For this review, use the dimensioned drawing (mm, ordinates from the lowest corner) and the shaded views. A direction names the side the tool comes from. Coordinates: 2 decimals unless noted, no trailing zeros. Order: outer loops, then holes, each group sorted by start corner. A loop starts at its lowest first (then second) coordinate and runs counter-clockwise, first axis right, second up. Notation, with made-up numbers: (63, 79) -> (107, 79) arc R21 ccw to (107, 105) -> close; hole circle Ø3 at (0, 56). An arc over 180 degrees is marked (long way). Use one line per item in the form item = value. Start each with the question number.
(1) For the marked faces 1, 2 and 3, list the 3-axis set-ups (+Z, -Z, +X, -X, +Y, -Y) from which the entire face can be reached by the end or side of a thin tool; tool diameter is ignored.
(2) Take a section at C-C (y = 513.5). State the section outline as (x, z) points.
(3) Take a section at A-A (x = 444.5). State the section outline as (y, z) points, then the cut area to 3 significant figures.
(4) Wall thickness on line 1 along Y through (x, z) = (448, 212); line 2 along Y through (x, z) = (1625, 26) (1 decimal); line 3 along X through (y, z) = (483.5, 214) (1 decimal): over which ranges is each line inside the solid? List them lowest first.
(5) Take a section at D-D (x = 1898.5). State the section outline as (y, z) points (1 decimal), then the cut area to 3 significant figures.
(6) Insertion check: pin 1 Ø1.5 at (x, z) = (999.5, 161.5) entering from +Y; pin 2 Ø10 at (y, z) = (686, 196.5) entering from -X; pin 3 Ø1 at (y, z) = (616.5, 172.5) entering from -X. Each pin has a flat end and moves straight along its axis. Give the tip position at first contact, or say it passes through.
(7) Mouldability with a two-part tool opening along X and no side actions: class the marked faces 4, 5 and 6 as +X half, -X half, draft (parallel to the pull), parting line (faces both ways), or undercut.
(8) Take a section at B-B (z = 207). State the section outline as (x, y) points (1 decimal), then the cut area to 3 significant figures.
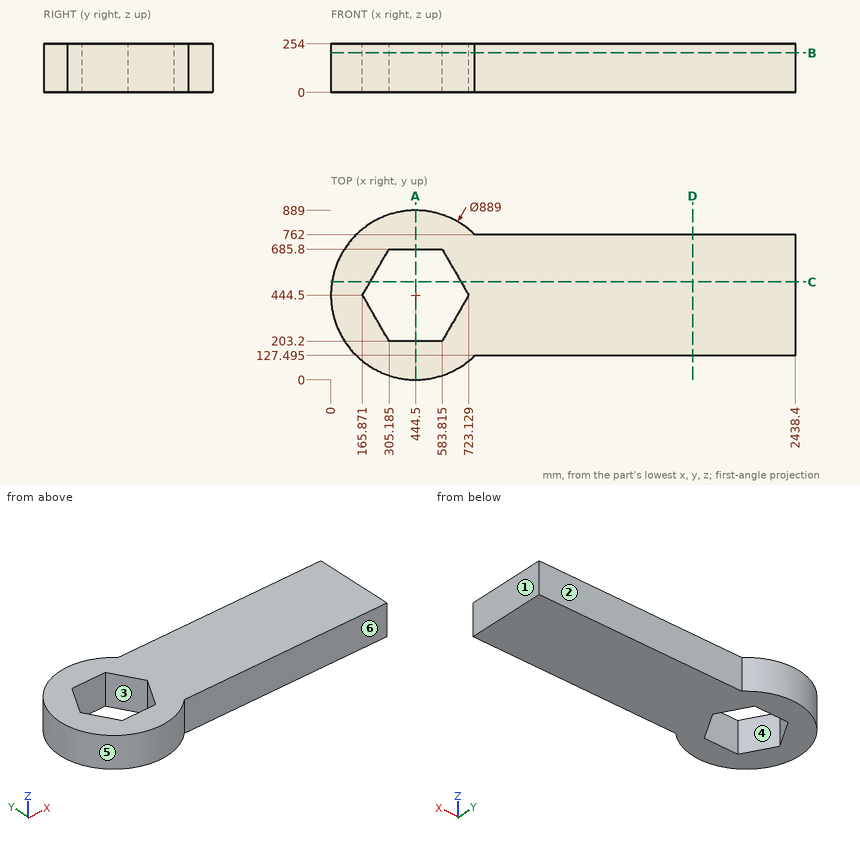
Findings:
q1.face_1 = +Z, -Z, +X, +Y, -Y
q1.face_2 = +Z, -Z, +X, +Y
q1.face_3 = +Z, -Z
q2.outline = (5.39, 0) -> (205.71, 0) -> (205.71, 254) -> (5.39, 254) -> close; (683.29, 0) -> (2438.4, 0) -> (2438.4, 254) -> (683.29, 254) -> close
q3.outline = (0, 0) -> (203.2, 0) -> (203.2, 254) -> (0, 254) -> close; (685.8, 0) -> (889, 0) -> (889, 254) -> (685.8, 254) -> close
q3.area = 103,000 mm²
q4.line_1 = 0.01 to 203.2, 685.8 to 888.99
q4.line_2 = 127.5 to 762
q4.line_3 = 1.7 to 188.4, 700.6 to 2438.4
q5.outline = (127.5, 0) -> (762, 0) -> (762, 254) -> (127.5, 254) -> close
q5.area = 161,000 mm²
q6.pin_1 = 762
q6.pin_2 = 68.14
q6.pin_3 = 34.42
q7.face_4 = undercut
q7.face_5 = parting line
q7.face_6 = draft
q8.outline = (755.6, 762) arc R444.5 ccw (long way) to (756.1, 127.5) -> (2438.4, 127.5) -> (2438.4, 762) -> close; hole (165.9, 444.5) -> (305.2, 203.2) -> (583.8, 203.2) -> (723.1, 444.5) -> (583.8, 685.8) -> (305.2, 685.8) -> close
q8.area = 1,430,000 mm²
